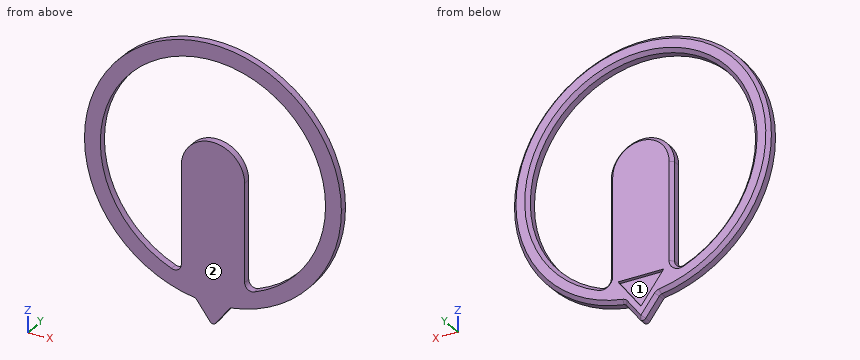
```python
from build123d import *

# Parameters (mm, degrees)
SKETCH2_R             = 0.786234884
BOSS_EXTRUDE1_DEPTH   = 0.3
SKETCH2_R_2           = 5.5
SKETCH2_R_3           = 3.2
BOSS_EXTRUDE1_2_DEPTH = 0.3
BOSS_EXTRUDE2_DEPTH   = 0.3
SKETCH4_R             = 5.5
CUT_EXTRUDE1_DEPTH    = 1.3
FILLET1_R             = 0.2
FILLET2_R             = 0.1
CHAMFER1_SIZE         = 0.1
CUT_EXTRUDE2_DEPTH    = 0.1


with BuildPart() as part:
    # Sketch2 → Boss-Extrude1 (new body)
    with BuildSketch(Plane(origin=(0, 0, 0), x_dir=(1, 0, 0), z_dir=(0, 1, 0))):
        Circle(SKETCH2_R)
    extrude(amount=BOSS_EXTRUDE1_DEPTH)



with BuildPart() as body_2:
    # Sketch2 → Boss-Extrude1 2 (new body)
    with BuildSketch(Plane(origin=(0, 0, 0), x_dir=(1, 0, 0), z_dir=(0, 1, 0))):
        Circle(SKETCH2_R_2)
        Circle(SKETCH2_R_3, mode=Mode.SUBTRACT)
    extrude(amount=BOSS_EXTRUDE1_2_DEPTH)


with BuildPart() as part_1:
    add(part.part)

    add(body_2.part)  # Boss-Extrude2 merges body 2
    # Sketch3 → Boss-Extrude2 (add)
    with BuildSketch(Plane(origin=(0, 0.3, 0), x_dir=(1, 0, 0), z_dir=(0, 1, 0))):
        with BuildLine():
            Line((-0.9, 0), (-0.9, 3.441526045))
            Line((-0.9, 3.441526045), (0.9, 3.441526045))
            Line((0.9, 3.441526045), (0.9, 0))
            ThreePointArc((0.9, 0), (0, -0.9), (-0.9, 0))
        make_face()
    extrude(amount=-BOSS_EXTRUDE2_DEPTH)

    # Sketch4 → Cut-Extrude1 (cut, through all)
    with BuildSketch(Plane(origin=(0, 0.3, 0), x_dir=(1, 0, 0), z_dir=(0, 1, 0))):
        Circle(SKETCH4_R)
        with BuildLine():
            ThreePointArc((3.65, 0), (-2.401287493, -2.748875839), (-0.490448426, 3.616899272))
            Line((-0.490448426, 3.616899272), (0, 4.270830507))
            Line((0, 4.270830507), (0.490448426, 3.616899272))
            ThreePointArc((0.490448426, 3.616899272), (2.748875839, 2.401287493), (3.65, 0))
        make_face(mode=Mode.SUBTRACT)
    extrude(amount=-CUT_EXTRUDE1_DEPTH, mode=Mode.SUBTRACT)

    # Fillet1
    fillet1_edges = [part_1.edges().sort_by_distance(p)[0] for p in [
        (-0.9, 0.15, -3.070830507),
        (0.9, 0.15, -3.070830507),
    ]]
    fillet(fillet1_edges, radius=FILLET1_R)

    # Fillet2
    fillet2_edges = [part_1.edges().sort_by_distance(p)[0] for p in [
        (0.490448426, 0.15, -3.616899272),
        (0, 0.15, -4.270830507),
        (-0.490448426, 0.15, -3.616899272),
    ]]
    fillet(fillet2_edges, radius=FILLET2_R)

    # Chamfer1
    chamfer1_edges = [part_1.edges().sort_by_distance(p)[0] for p in [
        (0, 0.3, 3.2),
        (-0.9, 0.3, -1.395528574),
        (0.987453713, 0.3, -2.956385104),
        (-0.987453713, 0.3, -2.956385104),
        (0, 0.3, 0.9),
        (0, 0.3, 3.65),
        (0.9, 0.3, -1.395528574),
        (0.272771923, 0.3, -3.907134609),
        (-0.272771923, 0.3, -3.907134609),
        (0, 0.3, -4.20416384),
        (0.494418226, 0.3, -3.624162542),
        (-0.494418226, 0.3, -3.624162542),
    ]]
    chamfer(chamfer1_edges, length=CHAMFER1_SIZE)

    # Sketch5 → Cut-Extrude2 (cut)
    with BuildSketch(Plane(origin=(0, 0.3, 0), x_dir=(1, 0, 0), z_dir=(0, 1, 0))):
        Polygon((-0.65, 2.987497173), (0.65, 2.987497173), (0, 3.85416384), align=None)
    extrude(amount=-CUT_EXTRUDE2_DEPTH, mode=Mode.SUBTRACT)


solid = part_1.part
```
Input: part model. Units: mm. Frame: model coordinates. Face numbers are marked on the shaded views. Coordinates: 2 decimals unless noted, no trailing zeros. Loops run counter-clockwise (first coordinate to the right, second up) from the corner with the lowest first, then second, coordinate; pieces in that order, holes last. Notation, with made-up numbers: M 54,10.25 L 81,10.25 A13 ccw 81,21.25 Z; hole C 65.5,-25.5 d5. An arc over 180 degrees is marked long. Answer in a Markdown table with one row per item.
1. Material intervals for line 1 (X direction, y = 0.15, z = 0); line 2 (Z direction, x = 0, y = 0.15); line 3 (Z direction, x = 1.75, y = 0.15), sorted ascending.
Response:
| item | result |
|---|---|
| line 1 | x = -3.65 to -3.2, -0.9 to 0.9, 3.2 to 3.65 |
| line 2 | z = -4.2 to 0.9, 3.2 to 3.65 |
| line 3 | z = -3.2 to -2.68, 2.68 to 3.2 |
2. Section A-A, the plane y = 0.15. Output: boundary loops of the cut face in (x, z).
Response:
| item | result |
|---|---|
| outline | M -0.53,-3.61 A0.1 cw -0.47,-3.65 L -0.08,-4.16 A0.1 ccw 0.08,-4.16 L 0.47,-3.65 A0.1 cw 0.53,-3.61 A3.65 ccw long Z; hole M -1.17,-2.98 A0.2 ccw -0.9,-2.79 L -0.9,0 A0.9 cw 0.9,0 L 0.9,-2.79 A0.2 ccw 1.17,-2.98 A3.2 ccw long Z |
3. Draft query along Z for the marked faces 1 and 2. Return one class per face: pulls with the +Z half, pulls with the -Z half, needs draft (parallel to the pull), parting line crosses it, or undercut.
Response:
| item | result |
|---|---|
| face 1 | undercut |
| face 2 | needs draft |
4. Section B-B, the plane z = -2.5. Count the separate pieces of the cut face and the enclosed holes in it, then the cut area to 3 significant figures.
Response:
| item | result |
|---|---|
| separate pieces | 3 |
| enclosed holes | 0 |
| area | 0.898 mm2 |
